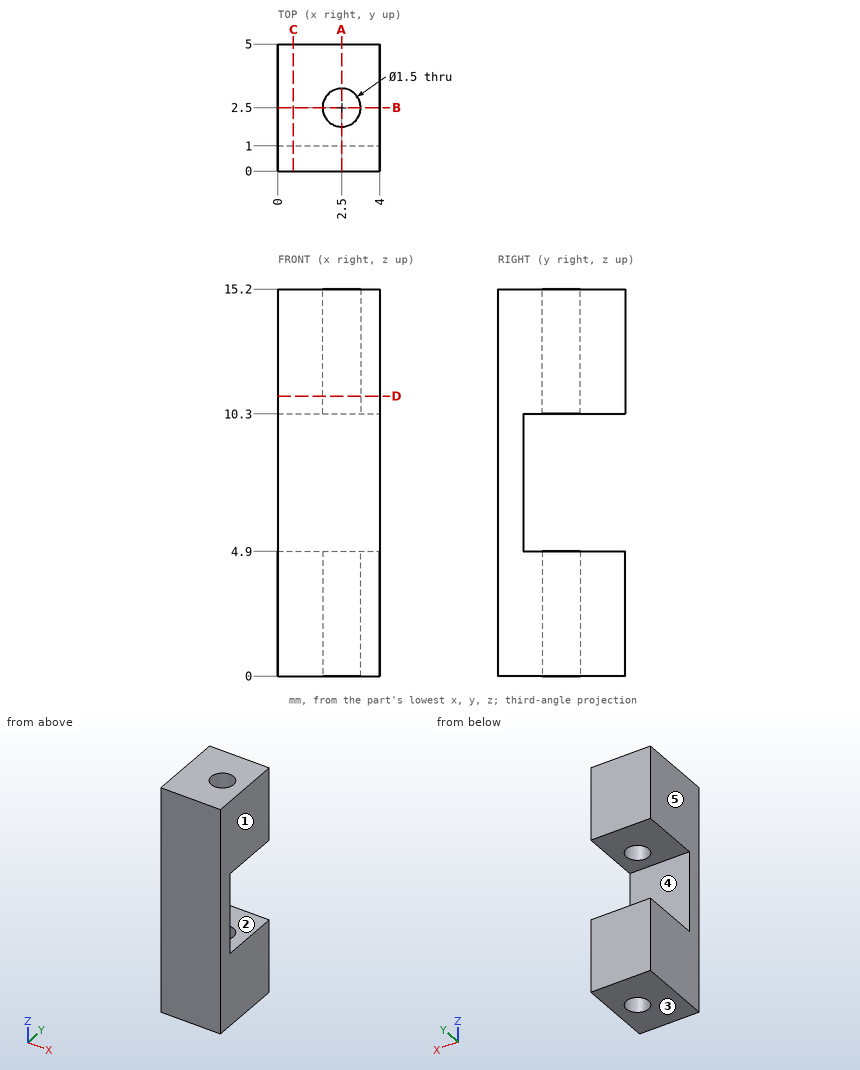
Geometry: see drawing. Coordinates: mm, zero at the bounding-box minimum. A direction names the side the tool comes from. Give positions to 0.01 mm unless a question says otherwise; leave off trailing zeros. Write each loop counter-clockwise with the first axis right and the second up, starting at its lowest first coordinate (ties: lowest second). Pieces come first, ordered by that corner, then holes. Notation, with made-up numbers: (27, 49.5) -> (35, 49.5) arc R25 ccw to (35, 86.5) -> close; hole circle Ø8 at (8, -28.75). An arc over 180 degrees is marked (long way). Use one line per item in the form item = value. Start each with the question number.
1) Section query D-D on z = 11. Return the cut outline in (x, y), then the cut area to 3 significant figures.
2) Set-up query: the marked faces 1 and 2. Return all of +Z, -Z, +X, -X, +Y, -Y with unobstructed straight access to the full face (end or side cutting, diameter ignored); none if empty.
3) Section query A-A on x = 2.5. Return the cut outline in (y, z).
4) Ray query, probe 1 along Y at (x, z) = (2.5, 14.2); probe 2 along Z at (x, y) = (3.05, 3.45); probe 3 along Y at (x, z) = (0.4, 5.5). Return the intervals inside material, ascending. Write a range as from..to.
5) Section query B-B on y = 2.5. Return the cut outline in (x, z).
6) Draft query along Z for the marked faces 3, 4 and 5. Return one class per face: pulls with the +Z half, pulls with the -Z half, needs draft (parallel to the pull), parting line crosses it, or undercut.
7) Pin query (flat end, axial travel): pin 1 (1.5 mm diameter, centred on y = 2, z = 1.5, fed in from -X); pin 2 (0.9 mm diameter, centred on x = 2.5, y = 2.5, fed in from +Z). Return the tip coordinate at first contact, or that it passes through.
8) Section query C-C on x = 0.6. Return the cut outline in (y, z), then the cut area to 3 significant figures.
Outcome:
q1.outline = (0, 0) -> (4, 0) -> (4, 5) -> (0, 5) -> close; hole circle Ø1.5 at (2.5, 2.5)
q1.area = 18.2 mm^2
q2.face_1 = +Z, -Z, +X, +Y, -Y
q2.face_2 = +X, -X, +Y
q3.outline = (0, 0) -> (1.75, 0) -> (1.75, 4.9) -> (1, 4.9) -> (1, 10.3) -> (1.75, 10.3) -> (1.75, 15.2) -> (0, 15.2) -> close; (3.25, 0) -> (5, 0) -> (5, 4.9) -> (3.25, 4.9) -> close; (3.25, 10.3) -> (5, 10.3) -> (5, 15.2) -> (3.25, 15.2) -> close
q4.probe_1 = 0..1.75, 3.25..5
q4.probe_2 = 0..4.9, 10.3..15.2
q4.probe_3 = 0..1
q5.outline = (0, 0) -> (1.75, 0) -> (1.75, 4.9) -> (0, 4.9) -> close; (0, 10.3) -> (1.75, 10.3) -> (1.75, 15.2) -> (0, 15.2) -> close; (3.25, 0) -> (4, 0) -> (4, 4.9) -> (3.25, 4.9) -> close; (3.25, 10.3) -> (4, 10.3) -> (4, 15.2) -> (3.25, 15.2) -> close
q6.face_3 = pulls with the -Z half
q6.face_4 = undercut
q6.face_5 = needs draft
q7.pin_1 = 0
q7.pin_2 = through
q8.outline = (0, 0) -> (5, 0) -> (5, 4.9) -> (1, 4.9) -> (1, 10.3) -> (5, 10.3) -> (5, 15.2) -> (0, 15.2) -> close
q8.area = 54.4 mm^2
